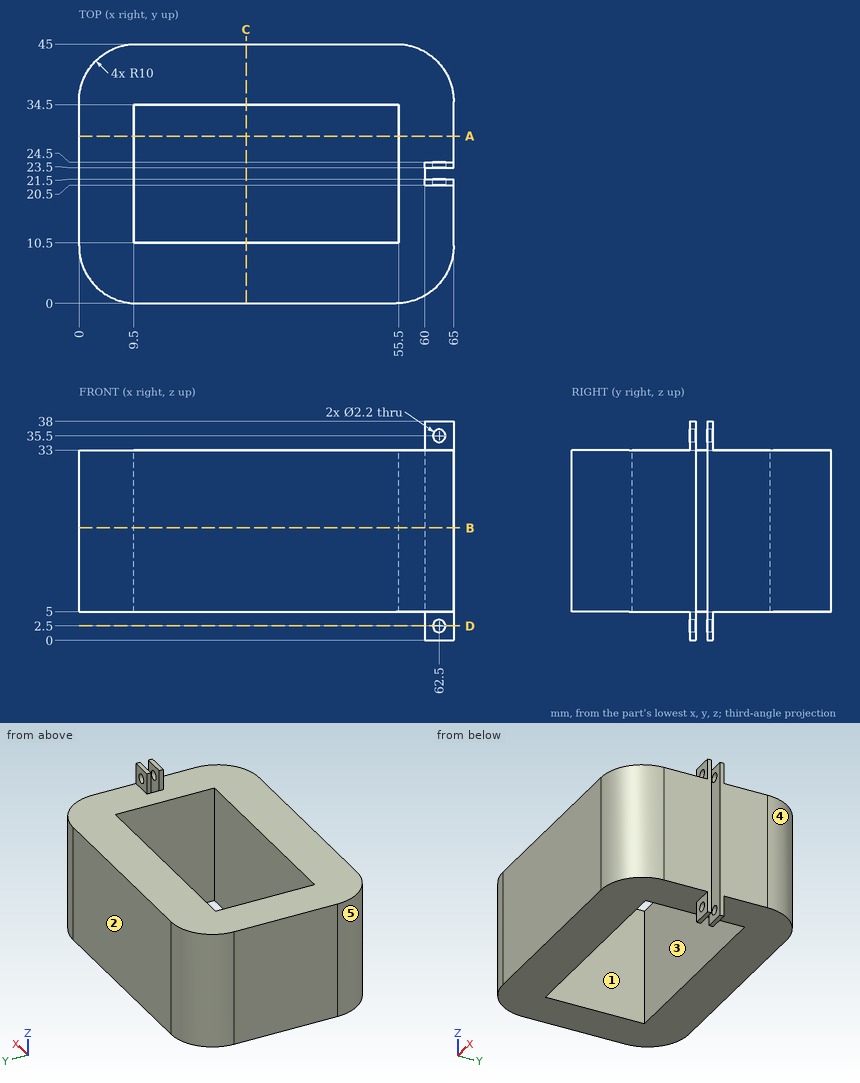
Geometry check sheet. Reference: drawing and pictorial views, mm from the part's lowest x, y, z. A direction names the side the tool comes from. Round coordinates to 2 decimals unless told otherwise and drop trailing zeros. Write each loop counter-clockwise with the first axis right and the second up, starting at its lowest first coordinate (ties: lowest second). Pieces come first, ordered by that corner, then holes. Notation, with made-up numbers: (-17, 41.25) -> (19, 41.25) arc R12 ccw to (19, 49.25) -> close; hole circle Ø9 at (71, 69.25). An arc over 180 degrees is marked (long way). Put each result on its own line as item: value.
1) Depth check by flat-ended pin: P1, Ø5.5, axis at x = 62, z = 3.5, coming from the -Y side; P2, Ø4, axis at x = 61.5, z = 18.5, coming from the +Y side; P3, Ø0.5, axis at y = 21, z = 35.5, coming from the -X side; P4, Ø1.3, axis at x = 62.5, z = 2.5, coming from the -Y side. Enter the tip coordinate at first touch or a pass-through.
Recorded:
P1: stops at y = 1.17
P2: stops at y = 43.93
P3: stops at x = 60
P4: passes through
2) Cross-section at A-A, the plane y = 29. Enter the section's corners in (x, z), plus the area to 3 significant figures.
Recorded:
outline: (0, 5) -> (9.5, 5) -> (9.5, 33) -> (0, 33) -> close; (55.5, 5) -> (65, 5) -> (65, 33) -> (55.5, 33) -> close
area: 532 mm2
3) Thickness scan on probe 1 along Z at (x, y) = (62.5, 24.2); probe 2 along Y at (x, z) = (39, 22); probe 3 along X at (y, z) = (29, 10). Record the ranges inside material, lowest first. Write a range as from..to.
Recorded:
probe 1: z = 0..1.4, 3.6..34.4, 36.6..38
probe 2: y = 0..10.5, 34.5..45
probe 3: x = 0..9.5, 55.5..65
4) Release check for a two-part mould opening along X. For the marked faces 3, 4 and 5 record: pulls with the +X half, pulls with the -X half, needs draft (parallel to the pull), parting line crosses it, or undercut.
Recorded:
face 3: undercut
face 4: pulls with the +X half
face 5: pulls with the -X half
5) Access from +Z, -Z, +X, -X, +Y, -Y to the whole of each face (thin tool, end or side, straight path). Record for the marked faces 1 and 2.
Recorded:
face 1: +Z, -Z
face 2: +Z, -Z, +X, -X, +Y
6) Cross-section at C-C, the plane x = 29. Enter the section's corners in (y, z).
Recorded:
outline: (0, 5) -> (10.5, 5) -> (10.5, 33) -> (0, 33) -> close; (34.5, 5) -> (45, 5) -> (45, 33) -> (34.5, 33) -> close
7) Cross-section at B-B, the plane z = 19.5. Enter the section's corners in (x, y).
Recorded:
outline: (0, 10) arc R10 ccw to (10, 0) -> (55, 0) arc R10 ccw to (65, 10) -> (65, 21.5) -> (60, 21.5) -> (60, 23.5) -> (65, 23.5) -> (65, 35) arc R10 ccw to (55, 45) -> (10, 45) arc R10 ccw to (0, 35) -> close; hole (9.5, 10.5) -> (55.5, 10.5) -> (55.5, 34.5) -> (9.5, 34.5) -> close
8) Cross-section at D-D, the plane z = 2.5. Enter the section's corners in (x, y), plus the area to 3 significant figures.
Recorded:
outline: (60, 20.5) -> (61.4, 20.5) -> (61.4, 21.5) -> (60, 21.5) -> close; (60, 23.5) -> (61.4, 23.5) -> (61.4, 24.5) -> (60, 24.5) -> close; (63.6, 20.5) -> (65, 20.5) -> (65, 21.5) -> (63.6, 21.5) -> close; (63.6, 23.5) -> (65, 23.5) -> (65, 24.5) -> (63.6, 24.5) -> close
area: 5.60 mm2
